```python
from build123d import *

# Parameters (mm, degrees)
ESBO_O4_R                  = 12.5
ESBO_O4_R_2                = 10
CORTE_EXTRUS_O1_DEPTH      = 22
CORTE_EXTRUS_O1_DEPTH_BACK = 23
ESBO_O5_R                  = 2.5


with BuildPart() as part:
    # Varredura1: sweep along a path in Esboço3
    with BuildLine(Plane(origin=(0, 0, 0), x_dir=(0, 0, -1), z_dir=(1, 0, 0))) as varredura1_path:
        Line((0, 0), (0, 15))
        ThreePointArc((0, 15), (4.393398282, 25.606601718), (15, 30))
        Line((15, 30), (30, 30))
    # Esboço4 → Varredura1 (sweep)
    with BuildSketch(Plane(origin=(0, 0, 0), x_dir=(1, 0, 0), z_dir=(0, 1, 0))):
        Circle(ESBO_O4_R)
        Circle(ESBO_O4_R_2, mode=Mode.SUBTRACT)
    sweep(path=varredura1_path.line)

    # Esboço5 → Corte-extrusão1 (cut, two sides: drawn at the far end of the back side and taken through both)
    with BuildSketch(Plane(origin=(0, 0, 0), x_dir=(0, 0, -1), z_dir=(1, 0, 0)).offset(-CORTE_EXTRUS_O1_DEPTH_BACK)):
        with Locations(Location((4.393398282, 25.606601718, 0), (0, 0, 325.914839644))):
            Circle(ESBO_O5_R)
    extrude(amount=CORTE_EXTRUS_O1_DEPTH + CORTE_EXTRUS_O1_DEPTH_BACK, mode=Mode.SUBTRACT)


solid = part.part
```
Source: CAD feature listing. Evaluate the final solid. Frame: model axes, mm. A direction names the side the tool comes from. Round coordinates to 2 decimals unless told otherwise and drop trailing zeros. Loops run counter-clockwise (first coordinate to the right, second up) from the corner with the lowest first, then second, coordinate; pieces in that order, holes last. Notation, with made-up numbers: M -33.75,47.5 L 11.25,47.5 A22 ccw 11.25,70.5 Z; hole C -29.75,74 d4. An arc over 180 degrees is marked long. Use a Markdown table: item, result. Add a question column.
1. Pull-direction query (Y, two-part tool) for faces 1 (the cylindrical face through (-11.111, 25.459, -1.898)), 2 (the cylindrical face through (-2.71, 42.203, -22.605)), 3 (the flat face through (10.2, 0, -0.1)), 4 (the cylindrical face through (11.923, 7.605, -3.755)); classes: +Y half, -Y half, draft (parallel to the pull), parting line (faces both ways), or undercut.
2. Ray query, line 1 along Y through (x, z) = (0, -25.75); line 2 along Z through (x, y) = (0, 3.5). Return the intervals inside material, ascending. Write a range as [from, to].
3. Set-up query: faces 5 (the cylindrical face through (-2.17, 39.76, -22.6)), 6 (the cylindrical face through (-2.17, 7.6, 9.76)), 7 (the flat face through (0.1, 40.2, -30)). Return all of +Z, -Z, +X, -X, +Y, -Y with unobstructed straight access to the full face (end or side cutting, diameter ignored); none if empty.
4. Cut plane C-C, the plane z = -18.5. Output: boundary loops of the cut face in (x, y), and give its area (3 significant figures).
5. Cut plane A-A, the plane x = 0. Output: boundary loops of the cut face in (y, z), and give its area (3 significant figures).
6. Cut plane B-B, the plane y = 11.5. Output: boundary loops of the cut face in (x, z), and give its area (3 significant figures).
7. Contact query for flat-ended pins moving along their axis: pin 1 (1.5 mm diameter, centred on x = 8.5, y = 29, fed in from +Z); pin 2 (2 mm diameter, centred on y = 13, z = 5, fed in from +X); pin 3 (4 mm diameter, centred on x = 7.5, z = -5.5, fed in from +Y). Output: stop coordinate, or through.
Solution:
| question | item | result |
|---|---|---|
| 1 | face 1 | undercut |
| 1 | face 2 | parting line |
| 1 | face 3 | -Y half |
| 1 | face 4 | draft |
| 2 | line 1 | y = [17.5, 20], [40, 42.5] |
| 2 | line 2 | z = [-12.5, -10], [10, 12.5] |
| 3 | face 5 | -Z |
| 3 | face 6 | -Y |
| 3 | face 7 | -Z, +X, -X, +Y, -Y |
| 4 | outline | C 0,30 d25; hole C 0,30 d20 |
| 4 | area | 177 mm2 |
| 5 | outline | M 0,-12.5 L 15,-12.5 A2.5 cw 17.5,-15 L 17.5,-30 L 20,-30 L 20,-15 A5 ccw 15,-10 L 0,-10 Z; M 0,10 L 15,10 A25 cw 40,-15 L 40,-30 L 42.5,-30 L 42.5,-15 A27.5 ccw 15,12.5 L 0,12.5 Z |
| 5 | area | 268 mm2 |
| 6 | outline | C 0,0 d25; hole C 0,0 d20 |
| 6 | area | 177 mm2 |
| 7 | pin 1 | stops at z = 5.64 |
| 7 | pin 2 | stops at x = 11.84 |
| 7 | pin 3 | stops at y = 39.67 |
